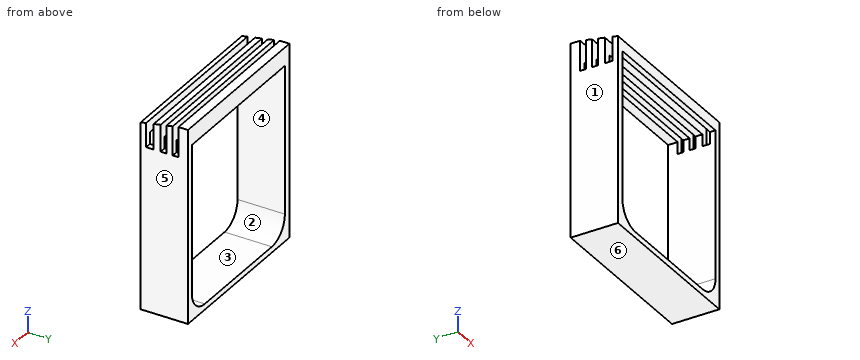
```python
from build123d import *

# Parameters (mm, degrees)
F0_W     = 780
F0_H     = 220
F1_DEPTH = 900
F2_W     = 715.66108
F2_H     = 788.264372
F3_DEPTH = 220
F5_DEPTH = 780
F6_W     = 780
F6_H     = 27.488791
F6_H_2   = 35.378739
F6_H_3   = 26.604801
F7_DEPTH = 140
F8_R     = 100


with BuildPart() as f1:
    # F0 (on Top) → F1 (new body)
    with BuildSketch(Plane.XY):
        with Locations((-390, 110)):
            Rectangle(F0_W, F0_H)
    extrude(amount=F1_DEPTH)

    # F2 (on face) → F3 (cut, through all)
    with BuildSketch(Plane.XZ):
        with Locations((-387.470587, 420.982849)):
            Rectangle(F2_W, F2_H)
    extrude(amount=-F3_DEPTH, mode=Mode.SUBTRACT)

    # F4 (on face) → F5 (cut, through all)
    with BuildSketch(Plane.YZ):
        Polygon((0, 867.352068), (175.820604, 900), (0, 900), align=None)
    extrude(amount=-F5_DEPTH, mode=Mode.SUBTRACT)

    # F6 (on face) → F7 (cut)
    with BuildSketch(Plane.XY.offset(900)):
        with Locations((-390, 106.569055)):
            Rectangle(F6_W, F6_H)
        with Locations((-390, 43.035474)):
            Rectangle(F6_W, F6_H_2)
        with Locations((-390, 162.518203)):
            Rectangle(F6_W, F6_H_3)
    extrude(amount=-F7_DEPTH, mode=Mode.SUBTRACT)

    # F8
    f8_edges = [f1.edges().sort_by_distance(p)[0] for p in [
        (-745.301127, 110, 26.850663),
        (-29.640047, 110, 26.850663),
    ]]
    fillet(f8_edges, radius=F8_R)


solid = f1.part
```
Part model, mm, in its own coordinate system. Face numbers are marked on the shaded views. A direction names the side the tool comes from. Round coordinates to 2 decimals unless told otherwise and drop trailing zeros. Loops run counter-clockwise (first coordinate to the right, second up) from the corner with the lowest first, then second, coordinate; pieces in that order, holes last. Notation, with made-up numbers: (31, 77.25) -> (60, 77.25) arc R14 ccw to (60, 82.25) -> close; hole circle Ø6 at (21.5, 82.5). An arc over 180 degrees is marked (long way). Use a Markdown table: item, result.
1) Drop flat-ended pins along their axis: pin 1 Ø20.5 at (x, y) = (-500.5, 14.5) entering from -Z; pin 2 Ø13.5 at (x, y) = (-13, 111.5) entering from +Z; pin 3 Ø12 at (x, z) = (-348.5, 809) entering from -Y. Give the stop position or say it passes through.
The answers:
| item | result |
|---|---|
| pin 1 | stops at z = 0 |
| pin 2 | stops at z = 760 |
| pin 3 | passes through |
2) Cut at A-A, the plane x = -542.5. List the corners of the cut face in (y, z).
The answers:
| item | result |
|---|---|
| outline | (0, 0) -> (220, 0) -> (220, 26.85) -> (0, 26.85) -> close; (0, 815.12) -> (25.35, 815.12) -> (25.35, 872.06) -> (0, 867.35) -> close; (60.72, 815.12) -> (92.82, 815.12) -> (92.82, 884.59) -> (60.72, 878.63) -> close; (120.31, 815.12) -> (149.22, 815.12) -> (149.22, 895.06) -> (120.31, 889.69) -> close; (175.82, 815.12) -> (220, 815.12) -> (220, 900) -> (175.82, 900) -> close |
3) Probe line 1 (Y direction, x = -144, z = 852); line 2 (X direction, y = 17, z = 384.5); line 3 (Z direction, x = -351.5, y = 148.5). List the from-to ranges inside material, lowest first. Write a range as [from, to].
The answers:
| item | result |
|---|---|
| line 1 | y = [0, 25.35], [60.72, 92.82], [120.31, 149.22], [175.82, 220] |
| line 2 | x = [-780, -745.3], [-29.64, 0] |
| line 3 | z = [0, 26.85], [815.12, 894.93] |
4) Cut at B-B, the plane z = 838. List the corners of the cut face in (x, y).
The answers:
| item | result |
|---|---|
| outline | (-780, 0) -> (0, 0) -> (0, 25.35) -> (-780, 25.35) -> close; (-780, 60.72) -> (0, 60.72) -> (0, 92.82) -> (-780, 92.82) -> close; (-780, 120.31) -> (0, 120.31) -> (0, 149.22) -> (-780, 149.22) -> close; (-780, 175.82) -> (0, 175.82) -> (0, 220) -> (-780, 220) -> close |
5) Tool access for the marked faces 1 and 2: list every direction of +Z, -Z, +X, -X, +Y, -Y with a clear straight run to the whole face (end or side of a thin tool).
The answers:
| item | result |
|---|---|
| face 1 | +Z, -Z, -X, +Y, -Y |
| face 2 | +Y, -Y |
6) Cut at D-D, the plane y = 39.5. List the corners of the cut face in (x, z).
The answers:
| item | result |
|---|---|
| outline | (-780, 0) -> (0, 0) -> (0, 760) -> (-29.64, 760) -> (-29.64, 126.85) arc R100 cw to (-129.64, 26.85) -> (-645.3, 26.85) arc R100 cw to (-745.3, 126.85) -> (-745.3, 760) -> (-780, 760) -> close |
7) Pull direction Z, two halves, no side cores. Call the marked faces 3, 4, 5 and 6: pulls with the +Z half, pulls with the -Z half, needs draft (parallel to the pull), parting line crosses it, or undercut.
The answers:
| item | result |
|---|---|
| face 3 | undercut |
| face 4 | undercut |
| face 5 | needs draft |
| face 6 | pulls with the -Z half |
8) Cut at C-C, the plane z = 327.5. List the corners of the cut face in (x, y).
The answers:
| item | result |
|---|---|
| outline | (-780, 0) -> (-745.3, 0) -> (-745.3, 220) -> (-780, 220) -> close; (-29.64, 0) -> (0, 0) -> (0, 220) -> (-29.64, 220) -> close |
